Drawing for the job (mm, zero at the part's lowest x, y, z). A direction names the side the tool comes from. Coordinates: 2 decimals unless noted, no trailing zeros. Loops run counter-clockwise (first coordinate to the right, second up) from the corner with the lowest first, then second, coordinate; pieces in that order, holes last. Notation, with made-up numbers: (41.5, 42.5) -> (95.5, 42.5) arc R28 cw to (95.5, 70.5) -> close; hole circle Ø10 at (87.5, -14.75). An arc over 180 degrees is marked (long way). Write item = value, one per line. Start each with the question number.
(1) Band-saw the part on C-C (y = 7.25). Count the separate pieces of the cut face and the enclosed holes in it, and give its area (3 significant figures).
(2) Band-saw the part on B-B (x = 8.5). Write the cut outline in (y, z).
(3) Pull direction X, two halves, no side cores. Call the marked faces 3, 4 and 5: +X half, -X half, draft (parallel to the pull), parting line (faces both ways), or undercut.
(4) Flat gauge pins, fed straight in: P1, Ø4, axis at y = 2, z = 4, coming from the -X side; P2, Ø2.5, axis at x = 2.49, z = 10.99, coming from the -Y side; P3, Ø6, axis at y = 8, z = 5, coming from the +X side (1 decimal); P4, Ø4, axis at y = 1, z = 7, coming from the -X side. Where does each tip first touch, or does it go through?
(5) Band-saw the part on D-D (x = 15). Write the cut outline in (y, z).
(6) Drill centre lines: line 1 (Z direction, x = 8.5, y = 9.15); line 2 (Z direction, x = 15.25, y = 9) (1 decimal); line 3 (Y direction, x = 8, z = 10.75). Where is each one in solid material? Low to high. Write a range as from..to.
(7) Tool access for the marked faces 1 and 2: list every direction of +Z, -Z, +X, -X, +Y, -Y with a clear straight run to the whole face (end or side of a thin tool).
(8) Band-saw the part on A-A (z = 8.5). Write the cut outline in (x, y).
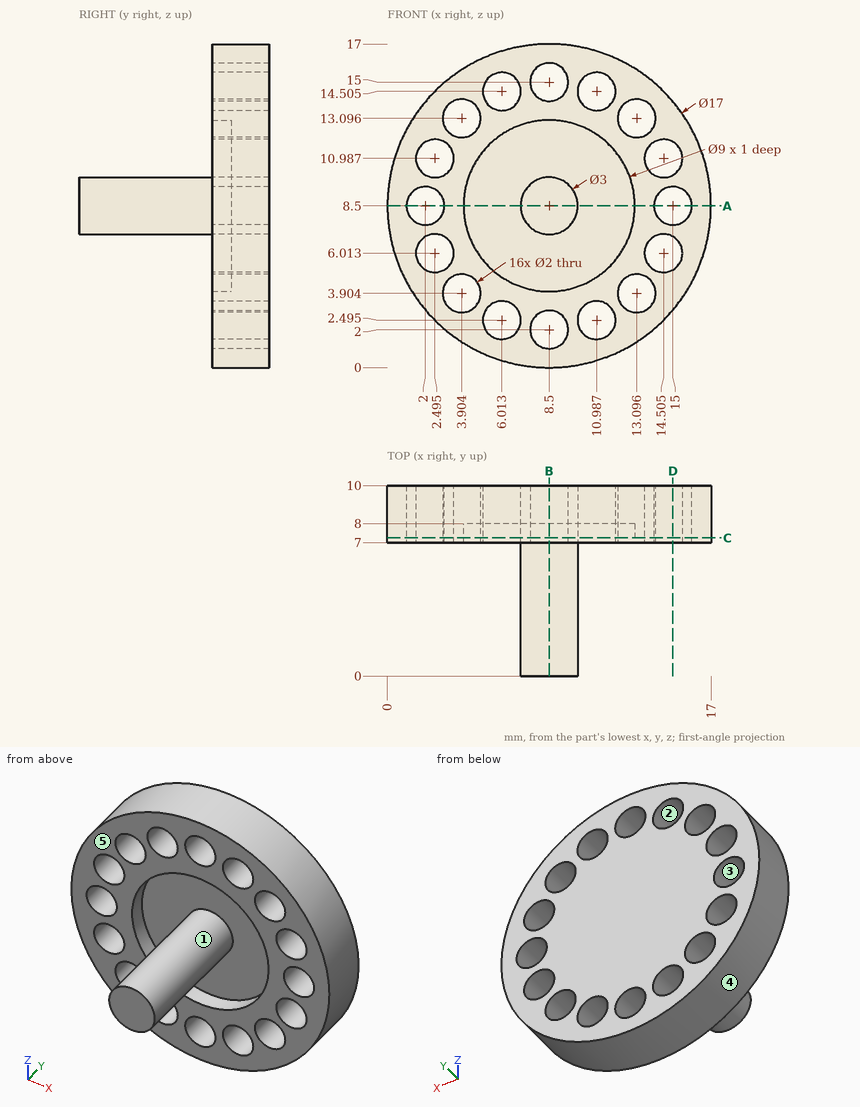
Findings below:
q1.separate_pieces = 2
q1.enclosed_holes = 17
q1.area = 120 mm²
q2.outline = (0, 7) -> (8, 7) -> (8, 4) -> (7, 4) -> (7, 3) -> (10, 3) -> (10, 14) -> (7, 14) -> (7, 13) -> (8, 13) -> (8, 10) -> (0, 10) -> close; (7, 0) -> (10, 0) -> (10, 1) -> (7, 1) -> close; (7, 16) -> (10, 16) -> (10, 17) -> (7, 17) -> close
q3.face_3 = undercut
q3.face_4 = parting line
q3.face_5 = draft
q4.P1 = through
q4.P2 = 7
q4.P3 = 17
q4.P4 = 7
q5.outline = (7, 3.02) -> (10, 3.02) -> (10, 5.14) -> (7, 5.14) -> close; (7, 6.88) -> (10, 6.88) -> (10, 7.5) -> (7, 7.5) -> close; (7, 9.5) -> (10, 9.5) -> (10, 10.12) -> (7, 10.12) -> close; (7, 11.86) -> (10, 11.86) -> (10, 13.98) -> (7, 13.98) -> close
q6.line_1 = 0..1, 3..14, 16..17
q6.line_2 = 3.3..5.3, 6.7..7.5, 9.5..10.3, 11.7..13.7
q6.line_3 = 8..10
q7.face_1 = -Y
q7.face_2 = +Y, -Y
q8.outline = (0, 7) -> (1, 7) -> (1, 10) -> (0, 10) -> close; (3, 7) -> (4, 7) -> (4, 8) -> (7, 8) -> (7, 0) -> (10, 0) -> (10, 8) -> (13, 8) -> (13, 7) -> (14, 7) -> (14, 10) -> (3, 10) -> close; (16, 7) -> (17, 7) -> (17, 10) -> (16, 10) -> close
